The model under review builds one solid part; all positions refer to its coordinate system, in mm. A direction names the side the tool comes from. Round coordinates to 2 decimals unless told otherwise and drop trailing zeros. Write each loop counter-clockwise with the first axis right and the second up, starting at its lowest first coordinate (ties: lowest second). Pieces come first, ordered by that corner, then holes. Notation, with made-up numbers: (-34, -38) - (-1, -38) arc R18 cw to (-1, -33) - close; hole circle Ø6 at (31, 78.25). An arc over 180 degrees is marked (long way). Return JSON: item names as keys, results as strings.
Autodesk Fusion 360 part; units mm, degrees
sketch "Sketch24" plane through (0, 0, 0) normal (0, 0, 1) x (1, 0, 0)
  line L0 (0, 0) -> (24, 0)
  line L1 (24, 0) -> (24, 18.5)
  line L2 (24, 18.5) -> (0, 18.5)
  line L3 (0, 18.5) -> (0, 0)
  dimension "d200" = 24
  dimension "d201" = 18.5
sketch "Sketch25" plane through (0, 0, 0) normal (0, 0, 1) x (1, 0, 0)
  line L0 (0, 0) -> (24, 0)
  line L1 (0, 18.5) -> (0, 0)
extrude "Extrude16" add sketch "Sketch24" along normal blind 3
sketch "Sketch26" plane through (0, 0, 3) normal (0, 0, 1) x (-1, 0, 0)
  line L0 (0, -18.5) -> (0, 0)
  line L1 (0, 0) -> (-24, 0)
  line L2 (-24, 0) -> (-24, -18.5)
  line L3 (-24, -18.5) -> (0, -18.5)
  point P0 (-3, -3)
  dimension "d206" = 3
  dimension "d207" = 3
hole "Hole7" at (3, 3, 3) direction (0, 0, -1) diameter 3.2 depth 3 tip angle 118
pattern_linear "R-Pattern3" count 2 spacing 18 along (1, 0, 0) count 2 spacing 12.5 along (0, 1, 0) of "Hole7"
sketch "Sketch27" plane through (0, 0, 0) normal (0, 0, 1) x (1, 0, 0)
  line L0 (-44, 10) -> (-30, 10)
  line L1 (-30, 10) -> (-30, 34)
  line L2 (-30, 34) -> (-44, 34)
  line L3 (-44, 34) -> (-44, 10) construction
  line L4 (-41.25, 37.25) -> (-32.75, 37.25)
  line L5 (-32.75, 37.25) -> (-32.75, 35.25)
  line L6 (-32.75, 35.25) -> (-41.25, 35.25)
  line L7 (-41.25, 35.25) -> (-41.25, 37.25)
  line L8 (-41.25, 8.75) -> (-32.75, 8.75)
  line L9 (-32.75, 8.75) -> (-32.75, 6.75)
  line L10 (-32.75, 6.75) -> (-41.25, 6.75)
  line L11 (-41.25, 6.75) -> (-41.25, 8.75)
  line L12 (-44, 34) -> (-44, 38.5)
  line L13 (-44, 38.5) -> (-27, 38.5)
  line L14 (-44, 10) -> (-44, 5.5)
  line L15 (-44, 5.5) -> (-27, 5.5)
  line L16 (-27, 5.5) -> (0, 0)
  line L17 (0, 0) -> (0, 18.5)
  line L18 (0, 18.5) -> (-27, 24)
  line L19 (-27, 24) -> (-27, 5.5) construction
  line L20 (-27, 38.5) -> (-27, 24)
  line L21 (-24, 18.2862) -> (-3, 14.0084)
  line L22 (-3, 14.0084) -> (-3, 5.7138)
  line L23 (-3, 5.7138) -> (-24, 9.9916)
  line L24 (-24, 9.9916) -> (-24, 18.2862)
  dimension "d215" = 14
  dimension "d216" = 24
  dimension "d217" = 30
  dimension "d218" = 10
  dimension "d219" = 8.5
  dimension "d220" = 2
  dimension "d221" = 2.75
  dimension "d222" = 1.25
  dimension "d223" = 8.5
  dimension "d224" = 2
  dimension "d225" = 2.75
  dimension "d226" = 1.25
  dimension "d227" = 4.5
  dimension "d228" = 17
  dimension "d229" = 4.5
  dimension "d230" = 17
  dimension "d231" = 18.5
  dimension "d232" = 3
  dimension "d233" = 3
  dimension "d235" = 5
  dimension "d236" = 5
extrude "Extrude17" add sketch "Sketch27" along normal blind 3
fillet "Fillet20" radius 1 2 edges at (24, 0, 1.5) (24, 18.5, 1.5)
fillet "Fillet21" radius 3 4 edges at (-24, 18.2862, 1.5) (-3, 14.0084, 1.5) (-3, 5.7138, 1.5) (-24, 9.9916, 1.5)
fillet "Fillet22" radius 5 4 edges at (0, 18.5, 1.5) (0, 0, 1.5) (-27, 5.5, 1.5) (-27, 24, 1.5)
fillet "Fillet23" radius 2 7 edges at (-44, 38.5, 1.5) (-44, 34, 1.5) (-44, 10, 1.5) (-44, 5.5, 1.5) (-27, 38.5, 1.5) (-30, 34, 1.5) (-30, 10, 1.5)
fillet "Fillet24" radius 1 8 edges at (-32.75, 37.25, 1.5) (-32.75, 35.25, 1.5) (-41.25, 35.25, 1.5) (-41.25, 37.25, 1.5) (-41.25, 8.75, 1.5) (-41.25, 6.75, 1.5) (-32.75, 6.75, 1.5) (-32.75, 8.75, 1.5)
sketch "Sketch28" plane through (0, 0, 3) normal (0, 0, 1) x (-1, 0, 0)
  arc A0 (27, -36.5) -> (29, -38.5) centre (29, -36.5) ccw
  line L0 (29, -38.5) -> (42, -38.5)
  arc A1 (42, -38.5) -> (44, -36.5) centre (42, -36.5) ccw
  line L1 (44, -36.5) -> (44, -36)
  arc A2 (44, -36) -> (42, -34) centre (42, -36) ccw
  line L2 (42, -34) -> (32, -34)
  arc A3 (30, -32) -> (32, -34) centre (32, -32) ccw
  line L3 (30, -32) -> (30, -12)
  arc A4 (32, -10) -> (30, -12) centre (32, -12) ccw
  line L4 (32, -10) -> (42, -10)
  arc A5 (42, -10) -> (44, -8) centre (42, -8) ccw
  line L5 (44, -8) -> (44, -7.5)
  arc A6 (44, -7.5) -> (42, -5.5) centre (42, -7.5) ccw
  line L6 (42, -5.5) -> (27.5041, -5.5)
  arc A7 (26.5061, -5.3994) -> (27.5041, -5.5) centre (27.5041, -0.5) ccw
  line L7 (26.5061, -5.3994) -> (0.4939, -0.1006)
  arc A8 (0.4939, -0.1006) -> (-0.5041, 0) centre (-0.5041, -5) ccw
  line L8 (-0.5041, 0) -> (-23, 0)
  arc A9 (-23, 0) -> (-24, -1) centre (-23, -1) ccw
  line L9 (-24, -1) -> (-24, -17.5)
  arc A10 (-24, -17.5) -> (-23, -18.5) centre (-23, -17.5) ccw
  line L10 (-23, -18.5) -> (-0.5041, -18.5)
  arc A11 (0.4939, -18.6006) -> (-0.5041, -18.5) centre (-0.5041, -23.5) ccw
  line L11 (0.4939, -18.6006) -> (22.998, -23.1848)
  arc A12 (27, -28.0842) -> (22.998, -23.1848) centre (22, -28.0842) ccw
  line L12 (27, -28.0842) -> (27, -36.5)
  line L13 (33.75, -6.75) -> (40.25, -6.75)
  arc A13 (40.25, -8.75) -> (40.25, -6.75) centre (40.25, -7.75) ccw
  line L14 (40.25, -8.75) -> (33.75, -8.75)
  arc A14 (33.75, -6.75) -> (33.75, -8.75) centre (33.75, -7.75) ccw
  line L15 (6.5988, -6.4469) -> (21.5988, -9.5024)
  arc A15 (24, -12.4421) -> (21.5988, -9.5024) centre (21, -12.4421) ccw
  line L16 (24, -12.4421) -> (24, -14.6135)
  arc A16 (20.4012, -17.5531) -> (24, -14.6135) centre (21, -14.6135) ccw
  line L17 (20.4012, -17.5531) -> (5.4012, -14.4976)
  arc A17 (3, -11.5579) -> (5.4012, -14.4976) centre (6, -11.5579) ccw
  line L18 (3, -11.5579) -> (3, -9.3865)
  arc A18 (6.5988, -6.4469) -> (3, -9.3865) centre (6, -9.3865) ccw
  line L19 (33.75, -35.25) -> (40.25, -35.25)
  arc A19 (41.25, -36.25) -> (40.25, -35.25) centre (40.25, -36.25) ccw
  arc A20 (40.25, -37.25) -> (41.25, -36.25) centre (40.25, -36.25) ccw
  line L20 (40.25, -37.25) -> (33.75, -37.25)
  arc A21 (32.75, -36.25) -> (33.75, -37.25) centre (33.75, -36.25) ccw
  arc A22 (33.75, -35.25) -> (32.75, -36.25) centre (33.75, -36.25) ccw
  circle A23 centre (-21, -15.5) radius 1.6
  circle A24 centre (-3, -15.5) radius 1.6
  circle A25 centre (-21, -3) radius 1.6
  circle A26 centre (-3, -3) radius 1.6
  circle A27 centre (-12, -9.25) radius 6
  point P0 (-12, -9.25)
  dimension "d249" = 12
  dimension "d250" = 9.25
  dimension "d251" = 12
extrude "Extrude18" cut sketch "Sketch28" against normal blind 3 contours A27
equation "d250 = ( 18.5 / 2 ) * 1 mm"
(1) Add section C-C (x = -18.5). Write out the cut boundary in (y, z), plus the area to 3 significant figures.
Filled in:
{"outline": "(3.77, 0) - (8.87, 0) - (8.87, 3) - (3.77, 3) - close; (17.17, 0) - (22.27, 0) - (22.27, 3) - (17.17, 3) - close", "area": "30.6 mm2"}
(2) Wall thickness on line 1 (Y direction, x = 3, z = 1.4); line 2 (Y direction, x = 12, z = 0.9); line 3 (Y direction, x = -32, z = 2.4): over which ranges is each line inside the solid? List them lowest first.
Filled in:
{"line 1": "y = 0 to 1.4, 4.6 to 13.9, 17.1 to 18.5", "line 2": "y = 0 to 3.25, 15.25 to 18.5", "line 3": "y = 5.5 to 10, 34 to 38.5"}
(3) Add section D-D (z = 1.3). Give the number of separate pieces and of enclosed holes in the cut face, plus the area to 3 significant figures.
Filled in:
{"separate pieces": "1", "enclosed holes": "8", "area": "826 mm2"}
(4) Clearance check with a flat-ended pin moving along its axis: pin 1 Ø1.5 at (x, z) = (-34.5, 2) entering from -Y. State where the tip first meets the part, or that it passes through.
Filled in:
{"pin 1": "stops at y = 5.5"}
(5) Mouldability with a two-part tool opening along X and no side actions: class faces 1 (the flat face through (-30, 22, 1)), 2 (the flat face through (-37, 34, 1)), 3 (the cylindrical face through (-27.57, 37.9, 1.52)), 4 (the flat face through (-37, 6.75, 1)) as released by +X, released by -X, zero draft, split by the parting line, or undercut.
Filled in:
{"face 1": "released by -X", "face 2": "zero draft", "face 3": "released by +X", "face 4": "undercut"}
(6) Add section B-B (y = 16). Write out the cut boundary in (x, z).
Filled in:
{"outline": "(-30, 0) - (-23.66, 0) - (-23.66, 3) - (-30, 3) - close; (-12.78, 0) - (1.48, 0) - (1.48, 3) - (-12.78, 3) - close; (4.52, 0) - (19.48, 0) - (19.48, 3) - (4.52, 3) - close; (22.52, 0) - (24, 0) - (24, 3) - (22.52, 3) - close"}
(7) For faces 5 (the flat face through (-13.006, 16.047, 1.479)), 6 (the flat face through (12, 18.5, 1)), 7 (the flat face through (-35, 5.5, 1)), list the 3-axis set-ups (+Z, -Z, +X, -X, +Y, -Y) from which the entire face can be reached by the end or side of a thin tool; tool diameter is ignored.
Filled in:
{"face 5": "+Z, -Z", "face 6": "+Z, -Z, +X, +Y", "face 7": "+Z, -Z, -X, -Y"}
(8) Add section A-A (x = 21). Write out the cut boundary in (y, z), plus the area to 3 significant figures.
Filled in:
{"outline": "(0, 0) - (1.4, 0) - (1.4, 3) - (0, 3) - close; (4.6, 0) - (13.9, 0) - (13.9, 3) - (4.6, 3) - close; (17.1, 0) - (18.5, 0) - (18.5, 3) - (17.1, 3) - close", "area": "36.3 mm2"}
